Check sheet for the modelled part. Datum: model origin and axes. Units: mm. Face numbers are marked on the shaded views. A direction names the side the tool comes from. Round coordinates to 2 decimals unless told otherwise and drop trailing zeros. Order: outer loops, then holes, each group sorted by start corner. A loop starts at its lowest first (then second) coordinate and runs counter-clockwise, first axis right, second up.
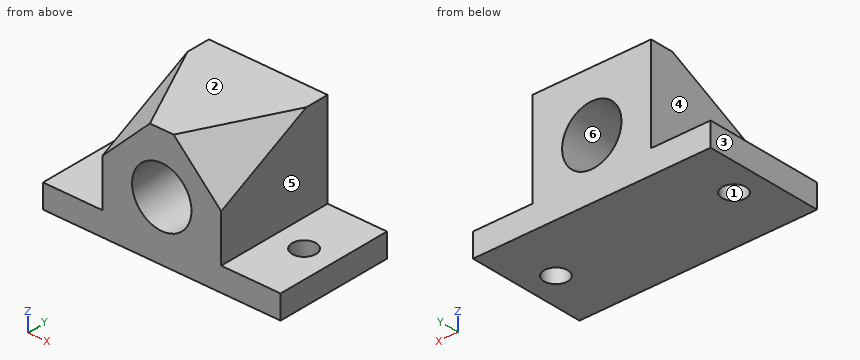
```python
from build123d import *

# Parameters (mm, degrees)
F0_W      = 100
F0_H      = 50
F1_DEPTH  = 50
F2_R      = 12.5
F3_DEPTH  = 50.001
F4_W      = 25
F4_H      = 40
F5_DEPTH  = 50.001
F6_R      = 5
F7_DEPTH  = 50.001
F12_W     = 63.2883179933
F12_H     = 65.7318904996
F13_DEPTH = 13.3333333333
F18_W     = 70.068154484
F18_H     = 62.6709284261
F19_DEPTH = 40


with BuildPart() as f1:
    # F0 (on Top) → F1 (new body)
    with BuildSketch(Plane.XY):
        Rectangle(F0_W, F0_H)
    extrude(amount=F1_DEPTH)

    # F2 (on face) → F3 (cut, through all)
    with BuildSketch(Plane.XZ.offset(25)):
        with Locations((0, 25)):
            Circle(F2_R)
    extrude(amount=-F3_DEPTH, mode=Mode.SUBTRACT)

    # F4 (on face) → F5 (cut, through all)
    with BuildSketch(Plane.XZ.offset(25)):
        with Locations((-37.5, 30)):
            Rectangle(F4_W, F4_H)
        with Locations((37.5, 30)):
            Rectangle(F4_W, F4_H)
    extrude(amount=-F5_DEPTH, mode=Mode.SUBTRACT)

    # F6 (on face) → F7 (cut, through all)
    with BuildSketch(Plane(origin=(0, 0, 0), x_dir=(1, 0, 0), z_dir=(0, 0, -1))):
        with Locations((-37.5, 0)):
            Circle(F6_R)
        with Locations((37.5, 0)):
            Circle(F6_R)
    extrude(amount=-F7_DEPTH, mode=Mode.SUBTRACT)

    # F12 (on plane+point) → F13 (cut, through all)
    with BuildSketch(Plane(origin=(38.8888888889, -19.4444444444, 38.8888888889), x_dir=(-0.2357022604, -0.9428090416, -0.2357022604), z_dir=(-0.6666666667, 0.3333333333, -0.6666666667))):
        with Locations((-9.0131862089, 14.5010352135)):
            Rectangle(F12_W, F12_H)
    extrude(amount=F13_DEPTH, mode=Mode.SUBTRACT)

    # F18 (on offset) → F19 (cut, through all)
    with BuildSketch(Plane(origin=(-56.6666666667, -28.3333333333, 56.6666666667), x_dir=(0.2357022604, -0.9428090416, -0.2357022604), z_dir=(-0.6666666667, -0.3333333333, 0.6666666667))):
        with Locations((-7.6787043363, 18.9961208962)):
            Rectangle(F18_W, F18_H)
    extrude(amount=-F19_DEPTH, mode=Mode.SUBTRACT)


solid = f1.part
```
Item 1: Scan lines: line 1 along Y through (x, z) = (37, 6); line 2 along X through (y, z) = (14, 38.5); line 3 along Z through (x, y) = (43, 22). Record each from-to range of solid material in increasing order.
Answer:
line 1: y = -25 to -4.97, 4.97 to 25
line 2: x = -25 to 25
line 3: z = 0 to 10
Item 2: Sectioned sample at B-B (x = 37.5). Record the cut outline in (y, z).
Answer:
outline: (-25, 0) - (-5, 0) - (-5, 10) - (-25, 10) - close; (5, 0) - (25, 0) - (25, 10) - (5, 10) - close
Item 3: Sectioned sample at D-D (y = -21.5). Record the cut outline in (x, z), and give its area (3 significant figures).
Answer:
outline: (-50, 0) - (50, 0) - (50, 10) - (25, 10) - (25, 31.75) - (6.75, 50) - (-6.75, 50) - (-25, 31.75) - (-25, 10) - (-50, 10) - close; hole circle Ø25 at (0, 25)
area: 2,180 mm2
Item 4: Sectioned sample at A-A (y = 0). Record the cut outline in (x, z), and give its area (3 significant figures).
Answer:
outline: (-50, 0) - (-42.5, 0) - (-42.5, 10) - (-50, 10) - close; (-32.5, 0) - (32.5, 0) - (32.5, 10) - (25, 10) - (25, 42.5) - (17.5, 50) - (-17.5, 50) - (-25, 42.5) - (-25, 10) - (-32.5, 10) - close; (42.5, 0) - (50, 0) - (50, 10) - (42.5, 10) - close; hole circle Ø25 at (0, 25)
area: 2,250 mm2
Item 5: Sectioned sample at C-C (z = 25). Record the cut outline in (x, y), and give its area (3 significant figures).
Answer:
outline: (-25, -25) - (-12.5, -25) - (-12.5, 25) - (-25, 25) - close; (12.5, -25) - (25, -25) - (25, 25) - (12.5, 25) - close
area: 1,250 mm2
Item 6: Go/stop test with flat-tipped pins: P1, Ø20, axis at x = -36, y = -2, coming from the +Z side; P2, Ø2, axis at y = -8, z = 16.5, coming from the +X side; P3, Ø6, axis at x = -37.5, y = 0, coming from the -Z side; P4, Ø1.5, axis at y = -13, z = 40.5, coming from the -X side. Record where each tip stops, or that it passes through.
Answer:
P1: stops at z = 10
P2: stops at x = 25
P3: passes through
P4: stops at x = -21.34
Item 7: Release check for a two-part mould opening along X. For the marked faces 1, 2 and 3 record: released by +X, released by -X, zero draft, split by the parting line, or undercut.
Answer:
face 1: undercut
face 2: zero draft
face 3: released by -X
Item 8: Access from +Z, -Z, +X, -X, +Y, -Y to the whole of each face (thin tool, end or side, straight path). Record for the marked faces 4, 5 and 6.
Answer:
face 4: +Z, -X, +Y, -Y
face 5: +Z, +X, +Y, -Y
face 6: +Y, -Y
